Read the model definition and answer for the solid it produces. Units are mm, in the model's axes. Face numbers are marked on the shaded views. A direction names the side the tool comes from. Round coordinates to 2 decimals unless told otherwise and drop trailing zeros. Order: outer loops, then holes, each group sorted by start corner. A loop starts at its lowest first (then second) coordinate and runs counter-clockwise, first axis right, second up. Notation, with made-up numbers: M 87.5,17 L 97.5,17 A15 ccw 97.5,29 Z; hole C 29.5,68 d4. An arc over 180 degrees is marked long. Use one line per item in the form item = value. Start each with the question number.
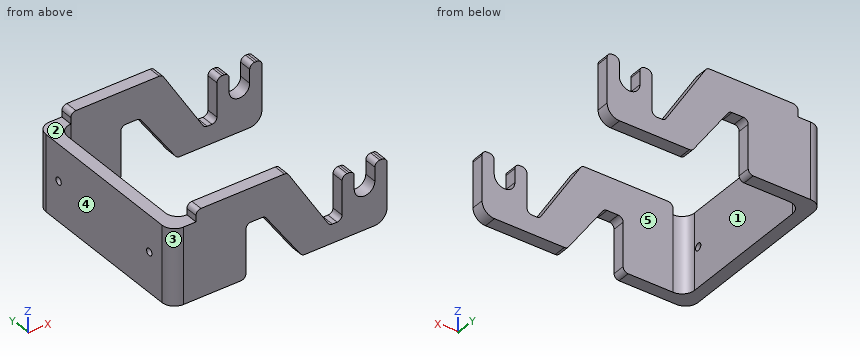
from build123d import *

# Parameters (mm, degrees)
PAD_DEPTH       = 35
SKETCH001_W     = 10
SKETCH001_H     = 4.5
POCKET_DEPTH    = 74.001
FILLET_R        = 2
FILLET001_R     = 5
SKETCH002_R     = 1.45
POCKET001_DEPTH = 5


with BuildPart() as part:
    # Sketch → Pad (new body)
    with BuildSketch(Plane.XY):
        Polygon((-43.25, 37), (43.25, 37), (43.25, 32), (-38.25, 32), (-38.25, -32), (43.25, -32), (43.25, -37), (-43.25, -37), align=None)
    extrude(amount=PAD_DEPTH)

    # Sketch001 → Pocket (cut, through all)
    with BuildSketch(Plane(origin=(0, 37, 0), x_dir=(-1, 0, 0), z_dir=(0, 1, 0))):
        with BuildLine():
            ThreePointArc((-38.375, 17.5), (-34.25, 13.375), (-30.125, 17.5))
            Line((-30.125, 17.5), (-30.125, 25))
            Line((-30.125, 25), (-25.25, 25))
            Line((-25.25, 25), (-25.25, 7.5))
            Line((-25.25, 7.5), (-20.25, 7.5))
            Line((-20.25, 7.5), (-3.25, 35))
            Line((-43.25, 35), (-3.25, 35))
            Line((-43.25, 25), (-43.25, 35))
            Line((-38.375, 25), (-43.25, 25))
            Line((-38.375, 17.5), (-38.375, 25))
        make_face()
        with Locations((38.25, 32.75)):
            Rectangle(SKETCH001_W, SKETCH001_H)
        Polygon((5.75, 21.5), (13.25, 21.5), (13.25, 0), (-9.25, 0), align=None)
    extrude(amount=-POCKET_DEPTH, mode=Mode.SUBTRACT)

    # Fillet
    fillet_edges = [part.edges().sort_by_distance(p)[0] for p in [
        (43.25, 34.5, 25),
        (38.375, 34.5, 25),
        (30.125, 34.5, 25),
        (25.25, 34.5, 25),
        (43.25, -34.5, 25),
        (38.375, -34.5, 25),
        (30.125, -34.5, 25),
        (25.25, -34.5, 25),
        (3.25, -34.5, 35),
        (-33.25, -34.5, 35),
        (-33.25, 34.5, 35),
        (3.25, 34.5, 35),
        (20.25, -34.5, 7.5),
        (20.25, 34.5, 7.5),
        (25.25, -34.5, 7.5),
        (25.25, 34.5, 7.5),
        (9.25, 34.5, 0),
        (9.25, -34.5, 0),
        (-5.75, -34.5, 21.5),
        (-5.75, 34.5, 21.5),
        (-13.25, 34.5, 0),
        (-13.25, -34.5, 0),
        (-13.25, 34.5, 21.5),
        (-13.25, -34.5, 21.5),
    ]]
    fillet(fillet_edges, radius=FILLET_R)

    # Fillet001
    fillet001_edges = [part.edges().sort_by_distance(p)[0] for p in [
        (43.25, 34.5, 0),
        (43.25, -34.5, 0),
        (-38.25, -32, 15.25),
        (-43.25, 37, 15.25),
        (-38.25, 32, 15.25),
        (-43.25, -37, 15.25),
    ]]
    fillet(fillet001_edges, radius=FILLET001_R)

    # Sketch002 → Pocket001 (cut)
    with BuildSketch(Plane(origin=(-43.25, 0, 0), x_dir=(0, -1, 0), z_dir=(-1, 0, 0))):
        with Locations((-25, 16)):
            Circle(SKETCH002_R)
        with Locations((25, 16)):
            Circle(SKETCH002_R)
    extrude(amount=-POCKET001_DEPTH, mode=Mode.SUBTRACT)


solid = part.part
Item 1: Find the intervals of material crossed by L1, parallel to Y at x = 4, z = 17.5; L2, parallel to Z at x = -39, y = -25; L3, parallel to X at y = 8, z = 7.5, in increasing order. Write a range as [from, to].
Item 2: Given P1, Ø4.5, axis at y = 25, z = 16, coming from the -X side; P2, Ø10, axis at x = 11.5, y = -26.5, coming from the +Z side; P3, Ø1.2, axis at y = 35, z = 31.5, coming from the -X side; P4, Ø1.3, axis at x = -8.5, y = -33.5, coming from the -Z side, each flat-ended and moving along its own axis, determine where each tip first touches the part or whether it passes through.
Item 3: Section B-B (y = -25) is taken. Write down the section's boundary in (x, z).
Item 4: Section C-C (z = 28.5) is taken. Write down the section's boundary in (x, y), and give its area (3 significant figures).
Item 5: Section A-A (x = -25) is taken. Write down the section's boundary in (y, z), and give its area (3 significant figures).
Item 6: A tool of negligible diameter and unlimited length cuts with its end or side. For the marked faces 4 and 5, from which of +Z, -Z, +X, -X, +Y, -Y can it reach the whole face along a straight path? Write none if from no direction.
Item 7: Section D-D (y = -15) is taken. Write down the section's boundary in (x, z).
Item 8: For a pull along Y with two mould halves and no side action, classify the marked faces 1, 2 and 3 as pulls with the +Y half, pulls with the -Y half, needs draft (parallel to the pull), parting line crosses it, or undercut.
The answers:
q1.L1 = [-37, -32], [32, 37]
q1.L2 = [0, 14.55], [17.45, 30.5]
q1.L3 = [-43.25, -38.25]
q2.P1 = -43.25
q2.P2 = through
q2.P3 = -33.25
q2.P4 = 21.5
q3.outline = M -43.25,0 L -38.25,0 L -38.25,14.55 L -43.25,14.55 Z; M -43.25,17.45 L -38.25,17.45 L -38.25,30.5 L -43.25,30.5 Z
q4.outline = M -43.25,-32 A5 ccw -38.25,-37 L 7.27,-37 L 7.27,-32 L -33.25,-32 A5 cw -38.25,-27 L -38.25,27 A5 cw -33.25,32 L 7.27,32 L 7.27,37 L -38.25,37 A5 ccw -43.25,32 Z
q4.area = 825 mm²
q5.outline = M -37,0 L -32,0 L -32,35 L -37,35 Z; M 32,0 L 37,0 L 37,35 L 32,35 Z
q5.area = 350 mm²
q6.face_4 = +Z, -Z, -X, +Y, -Y
q6.face_5 = +Z, -Z, +X
q7.outline = M -43.25,0 L -38.25,0 L -38.25,30.5 L -43.25,30.5 Z
q8.face_1 = undercut
q8.face_2 = needs draft
q8.face_3 = pulls with the -Y half
